Study the drawing (mm; zero at the part's minimum x, y, z) and answer. Give positions to 0.01 mm unless a question says otherwise; leave off trailing zeros. Order: outer loops, then holes, each group sorted by start corner. A loop starts at its lowest first (then second) coordinate and runs counter-clockwise, first axis right, second up. Notation, with made-up numbers: (-4, -10) - (47, -10) arc R25 cw to (47, 6) - close; hole circle Ø1 at (64, -5.5). An arc over 180 degrees is marked (long way). Write each question's results on one line, items separated by ' | '. Start each with the question number.
1. Section B-B (x = 84) is taken. Give the vertices of the cut face in (y, z) (1 decimal), and give its area (3 significant figures).
2. Section A-A (z = 33) is taken. Give the vertices of the cut face in (x, y) (1 decimal).
3. Flat-ended cylindrical pins translate along their axes: pin 1 (8 mm diameter, centred on y = 35.5, z = 17.5, fed in from -X); pin 2 (8 mm diameter, centred on y = 66.5, z = 92, fed in from -X); pin 3 (3 mm diameter, centred on y = 132.5, z = 35.5, fed in from -X). Find the tip coordinate at first contact, or state that the pin passes through.
4. Find the intervals of material crossed by L1, parallel to Y at x = 57.5, z = 7 (1 decimal); L2, parallel to Y at x = 25, z = 41 (1 decimal); L3, parallel to X at y = 187, z = 110, in increasing order.
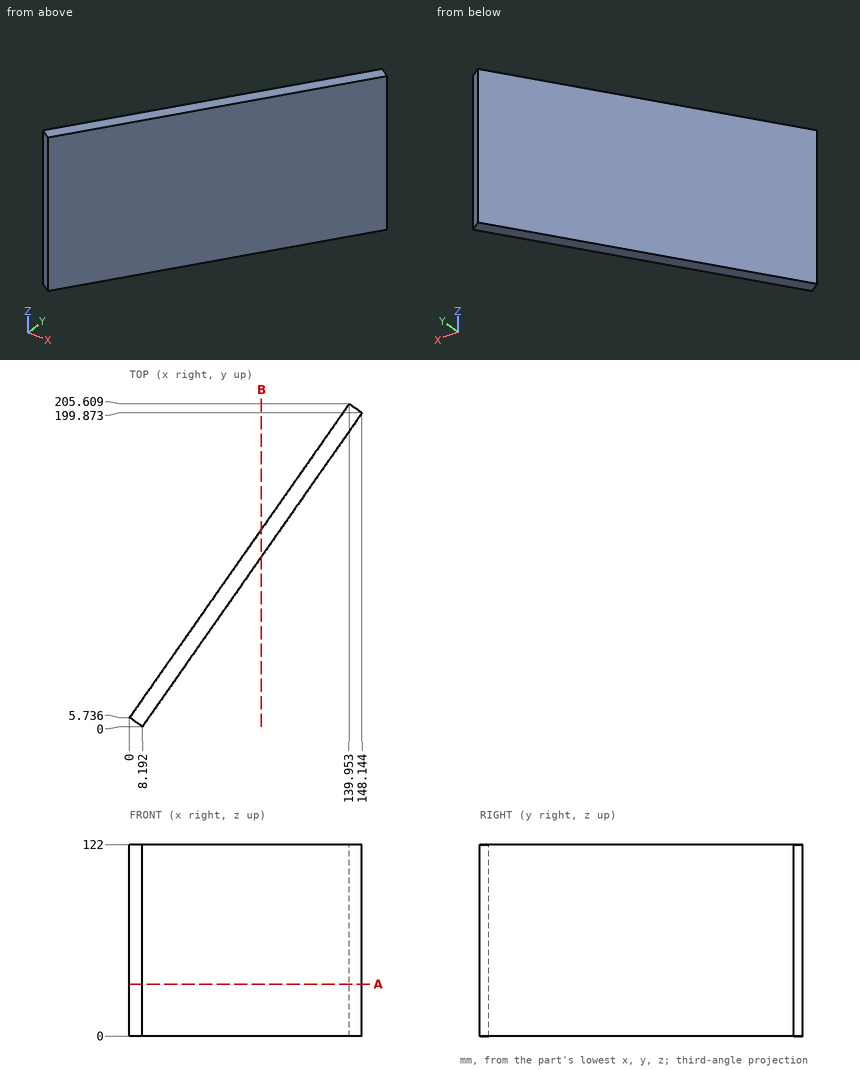
Reported:
1) outline: (108.3, 0) - (125.7, 0) - (125.7, 122) - (108.3, 122) - close | area: 2,130 mm²
2) outline: (0, 5.7) - (8.2, 0) - (148.1, 199.9) - (140, 205.6) - close
3) pin 1: x = 18.04 | pin 2: x = 39.75 | pin 3: x = 87.71
4) L1: 70.4 to 87.9 | L2: 24 to 41.4 | L3: 126.92 to 139.13
